Could you check a few things on this model? Use its own coordinates, in mm. Give positions to 0.01 mm unless a question says otherwise; leave off trailing zeros. Loops run counter-clockwise (first coordinate to the right, second up) from the corner with the lowest first, then second, coordinate; pieces in that order, holes last. Notation, with made-up numbers: M 77,58.25 L 122,58.25 A30 ccw 122,91.25 Z; hole C -24.5,54.5 d1. An arc over 180 degrees is marked long. Use a Markdown table: item, result. Add a question column.
1) Suppose I cut it at D-D on x = 185.5. List the corners of the cut face in (y, z) for me.
2) Suppose I cut it at C-C on y = 7.5. List the corners of the cut face in (x, z) for me, and give its area (3 significant figures).
3) Suppose I cut it at A-A on y = 35. List the corners of the cut face in (x, z) for me, and give its area (3 significant figures).
4) If I drill on line 1 along X through (y, z) = (45.5, 43); line 2 along Y through (x, z) = (17, 92.5); line 3 along Y through (x, z) = (174.5, -107), over which ranges is the centre line in solid material (lowest first)? Write a range as [from, to].
5) Suppose I cut it at B-B on z = -40.5. List the corners of the cut face in (x, y) for me, and give its area (3 significant figures).
6) We'd pull the mould along X, two halves only. Please class faces 1 (the cylindrical face through (-347.773, 45.502, 1.68)), 2 (the cylindrical face through (347.773, 45.502, 1.68)), 3 (the flat face through (5, 3, -120)): +X half, -X half, draft (parallel to the pull), parting line (faces both ways), or undercut.
7) Will these pins go through, and if not, where does the flat tip stop? pin 1 Ø6 at (y, z) = (23.5, -30.5) entering from +X; pin 2 Ø3 at (y, z) = (31, 47) entering from +X; pin 3 Ø10 at (y, z) = (-14, -85) entering from +X; pin 4 Ø10 at (y, z) = (7.5, -77) entering from -X.
```python
from build123d import *

# Parameters (mm, degrees)
AUFSATZ_LINEAR_AUSTRAGEN1_DEPTH = 120


with BuildPart() as part:
    # Skizze1 → Aufsatz-Linear austragen1 (new body, symmetric)
    with BuildSketch(Plane.XY):
        with BuildLine():
            Line((0, -15), (0, 45))
            ThreePointArc((0, 45), (-103.311330917, 38.513471526), (-205, 19.155766915))
            ThreePointArc((-205, 19.155766915), (-266.956521007, 18.203003185), (-322.60257584, 45.461668516))
            ThreePointArc((-322.60257584, 45.461668516), (-348.070218627, 45.253218096), (-352.237448898, 20.127962424))
            ThreePointArc((-352.237448898, 20.127962424), (-338.919122298, 1.513284408), (-322.60257584, -14.538331484))
            ThreePointArc((-322.60257584, -14.538331484), (-266.956521007, -41.796996815), (-205, -40.844233085))
            ThreePointArc((-205, -40.844233085), (-103.311330917, -21.486528474), (0, -15))
        make_face()
    aufsatz_linear_austragen1 = extrude(amount=AUFSATZ_LINEAR_AUSTRAGEN1_DEPTH, both=True)

    # Spiegeln1: Aufsatz-Linear austragen1 across plane
    add(aufsatz_linear_austragen1.mirror(Plane(origin=(0, 0, 120), x_dir=(0, 0, 1), z_dir=(1, 0, 0))))


solid = part.part
```
Answer block:
| question | item | result |
|---|---|---|
| 1 | outline | M -36.1,-120 L 23.9,-120 L 23.9,120 L -36.1,120 Z |
| 2 | outline | M -343.74,-120 L 343.74,-120 L 343.74,120 L -343.74,120 Z |
| 2 | area | 165,000 mm^2 |
| 3 | outline | M -354.41,-120 L -308.05,-120 L -308.05,120 L -354.41,120 Z; M -128.14,-120 L 128.14,-120 L 128.14,120 L -128.14,120 Z; M 308.05,-120 L 354.41,-120 L 354.41,120 L 308.05,120 Z |
| 3 | area | 83,800 mm^2 |
| 4 | line 1 | x = [-347.78, -322.65], [322.65, 347.78] |
| 4 | line 2 | y = [-15.17, 44.83] |
| 4 | line 3 | y = [-33.64, 26.36] |
| 5 | outline | M -352.24,20.13 A132.82 ccw -205,-40.84 A825.97 cw 205,-40.84 A132.82 ccw 352.24,20.13 A19.79 ccw 322.6,45.46 A132.82 cw 205,19.16 A825.97 ccw -205,19.16 A132.82 cw -322.6,45.46 A19.79 ccw Z |
| 5 | area | 41,600 mm^2 |
| 6 | face 1 | undercut |
| 6 | face 2 | undercut |
| 6 | face 3 | draft |
| 7 | pin 1 | stops at x = 354.65 |
| 7 | pin 2 | stops at x = 355 |
| 7 | pin 3 | stops at x = 328.89 |
| 7 | pin 4 | stops at x = -347.36 |
